from build123d import *

# Parameters (mm, degrees)
SKETCH1_W           = 50
SKETCH1_H           = 42
BOSS_EXTRUDE1_DEPTH = 3
SKETCH2_W           = 3
SKETCH2_H           = 42
BOSS_EXTRUDE2_DEPTH = 42
CUT_EXTRUDE2_DEPTH  = 10
SKETCH5_R           = 12.25
SKETCH5_R_2         = 1.25
CUT_EXTRUDE3_DEPTH  = 10


with BuildPart() as part:
    # Sketch1 → Boss-Extrude1 (new body)
    with BuildSketch(Plane(origin=(0, 0, 0), x_dir=(1, 0, 0), z_dir=(0, 1, 0))):
        Rectangle(SKETCH1_W, SKETCH1_H)
    extrude(amount=BOSS_EXTRUDE1_DEPTH)

    # Sketch2 → Boss-Extrude2 (add)
    with BuildSketch(Plane(origin=(0, 3, 0), x_dir=(1, 0, 0), z_dir=(0, 1, 0))):
        with Locations((-23.5, 0)):
            Rectangle(SKETCH2_W, SKETCH2_H)
    extrude(amount=BOSS_EXTRUDE2_DEPTH)

    # Sketch4 → Cut-Extrude2 (cut)
    with BuildSketch(Plane.ZY.offset(25)):
        with BuildLine():
            ThreePointArc((-8, 7.5), (-11, 10.5), (-14, 7.5))
            Line((-14, 7.5), (-8, 7.5))
        make_face()
        with BuildLine():
            Line((-8, 7.5), (-14, 7.5))
            ThreePointArc((-14, 7.5), (-11, 4.5), (-8, 7.5))
        make_face()
        with BuildLine():
            Line((-14, 37.5), (-14, 7.5))
            ThreePointArc((-14, 7.5), (-11, 10.5), (-8, 7.5))
            Line((-8, 7.5), (-8, 37.5))
            ThreePointArc((-8, 37.5), (-11, 34.5), (-14, 37.5))
        make_face()
        with BuildLine():
            ThreePointArc((-8, 37.5), (-11, 40.5), (-14, 37.5))
            Line((-14, 37.5), (-8, 37.5))
        make_face()
        with BuildLine():
            Line((-8, 37.5), (-14, 37.5))
            ThreePointArc((-14, 37.5), (-11, 34.5), (-8, 37.5))
        make_face()
        with BuildLine():
            Line((8, 37.5), (8, 7.5))
            ThreePointArc((8, 7.5), (11, 10.5), (14, 7.5))
            Line((14, 7.5), (14, 37.5))
            ThreePointArc((14, 37.5), (11, 34.5), (8, 37.5))
        make_face()
        with BuildLine():
            ThreePointArc((14, 37.5), (11, 40.5), (8, 37.5))
            Line((8, 37.5), (14, 37.5))
        make_face()
        with BuildLine():
            Line((14, 37.5), (8, 37.5))
            ThreePointArc((8, 37.5), (11, 34.5), (14, 37.5))
        make_face()
        with BuildLine():
            ThreePointArc((14, 7.5), (11, 10.5), (8, 7.5))
            Line((8, 7.5), (14, 7.5))
        make_face()
        with BuildLine():
            Line((14, 7.5), (8, 7.5))
            ThreePointArc((8, 7.5), (11, 4.5), (14, 7.5))
        make_face()
    extrude(amount=-CUT_EXTRUDE2_DEPTH, mode=Mode.SUBTRACT)

    # Sketch5 → Cut-Extrude3 (cut)
    with BuildSketch(Plane(origin=(0, 3, 0), x_dir=(1, 0, 0), z_dir=(0, 1, 0))):
        with Locations((4, 0)):
            Circle(SKETCH5_R)
        with Locations((-11.5, -15.5)):
            Circle(SKETCH5_R_2)
        with Locations((19.5, -15.5)):
            Circle(SKETCH5_R_2)
        with Locations((19.5, 15.5)):
            Circle(SKETCH5_R_2)
        with Locations((-11.5, 15.5)):
            Circle(SKETCH5_R_2)
    extrude(amount=-CUT_EXTRUDE3_DEPTH, mode=Mode.SUBTRACT)


solid = part.part
Work out the finished part from the listing and answer in its coordinate system (mm). A direction names the side the tool comes from. Coordinates: 2 decimals unless noted, no trailing zeros. Write each loop counter-clockwise with the first axis right and the second up, starting at its lowest first coordinate (ties: lowest second). Pieces come first, ordered by that corner, then holes. Notation, with made-up numbers: M 46,64 L 73,64 A31 cw 73,99 Z; hole C -26.75,21.25 d8. An arc over 180 degrees is marked long. Use one line per item in the form item = value. Start each with the question number.
1. Each of these flat-tipped pins is pushed along its axis until it touches: P1, Ø1.5, axis at x = 19.5, z = 15.5, coming from the -Y side; P2, Ø3, axis at x = 6, z = 13.5, coming from the -Y side; P3, Ø12, axis at y = 26.5, z = 12.5, coming from the +X side; P4, Ø3, axis at x = 19.5, z = -15.5, coming from the +Y side. Where does it stop, or does it pass through?
2. Straight lines are drawn through the part: probe 1 along X at (y, z) = (0.7, 15.5); probe 2 along Z at (x, y) = (-11.5, 0.7); probe 3 along Z at (x, y) = (19, 1). For each, find the intervals that lie inside material, in ascending order. Write a range as from..to.
3. The part is cut by section C-C (y = 18.5). Give the vertices of the cut face in (x, z).
4. The part is cut by section D-D (x = -11.5). Give the vertices of the cut face in (y, z), plus the area to 3 significant figures.
5. A tool of negligible diameter and unlimited length cuts with its end or side. For faces 1 (the face through (-22, 24, 0)), 2 (the face through (-25, 22, 0)), 3 (the face through (-23.5, 40.5, -10.9)), from which of +Z, -Z, +X, -X, +Y, -Y can it reach the whole face along a straight path? Write none if from no direction.
6. The part is cut by section A-A (z = -15.5). Give the vertices of the cut face in (x, y), plus the area to 3 significant figures.
7. The mould has two halves that part along X. Classify faces 4 (the face through (25, 1, 0)), 5 (the face through (-12.421, 1.521, 14.655)), 6 (the face through (-24, 22, 14)), 7 (the face through (20.172, 1.521, -16.554)): released by +X, released by -X, zero draft, split by the parting line, or undercut.
8. The part is cut by section B-B (x = 4). Give the vertices of the cut face in (y, z), plus the area to 3 significant figures.
Evaluation:
q1.P1 = through
q1.P2 = 0
q1.P3 = -22
q1.P4 = 3
q2.probe_1 = -25..-12.75, -10.25..18.25, 20.75..25
q2.probe_2 = -21..-16.75, -14.25..14.25, 16.75..21
q2.probe_3 = -21..-16.65, -14.35..14.35, 16.65..21
q3.outline = M -25,-21 L -22,-21 L -22,-14 L -25,-14 Z; M -25,-8 L -22,-8 L -22,8 L -25,8 Z; M -25,14 L -22,14 L -22,21 L -25,21 Z
q4.outline = M 0,-21 L 3,-21 L 3,-16.75 L 0,-16.75 Z; M 0,-14.25 L 3,-14.25 L 3,14.25 L 0,14.25 Z; M 0,16.75 L 3,16.75 L 3,21 L 0,21 Z
q4.area = 111 mm^2
q5.face_1 = +Z, -Z, +X, +Y
q5.face_2 = +Z, -Z, -X, +Y, -Y
q5.face_3 = +X, -X
q6.outline = M -25,0 L -12.75,0 L -12.75,3 L -22,3 L -22,45 L -25,45 Z; M -10.25,0 L 18.25,0 L 18.25,3 L -10.25,3 Z; M 20.75,0 L 25,0 L 25,3 L 20.75,3 Z
q6.area = 261 mm^2
q7.face_4 = released by +X
q7.face_5 = undercut
q7.face_6 = zero draft
q7.face_7 = undercut
q8.outline = M 0,-21 L 3,-21 L 3,-12.25 L 0,-12.25 Z; M 0,12.25 L 3,12.25 L 3,21 L 0,21 Z
q8.area = 52.5 mm^2
